```python
from build123d import *

# Parameters (mm, degrees)
SKETCH_W              = 18.5
SKETCH_H              = 18.5
SKETCH_R              = 8.15
PAD_DEPTH             = 4
SKETCH001_W           = 18.5
SKETCH001_H           = 18.5
PAD001_DEPTH          = 3
SKETCH002_R           = 9.25
SKETCH003_R           = 5.4
SKETCH005_R           = 5.4
PAD002_DEPTH          = 2
CHAMFER_SIZE          = 1.5
CHAMFER001_SIZE       = 1.5
POCKET_DEPTH          = 99.630527
POLARPATTERN_COUNT    = 4
SKETCH007_R           = 4.4
SKETCH008_R           = 5.4
SKETCH009_R           = 5.4
PAD003_DEPTH          = 7
SKETCH010_R           = 4.4
POCKET001_DEPTH       = 3
SKETCH011_W           = 1.7
SKETCH011_H           = 3
POCKET002_DEPTH       = 114.093887
POLARPATTERN001_COUNT = 5


with BuildPart() as part:
    # Sketch → Pad (new body)
    with BuildSketch(Plane.XY):
        Rectangle(SKETCH_W, SKETCH_H)
        Circle(SKETCH_R, mode=Mode.SUBTRACT)
    extrude(amount=PAD_DEPTH)

    # Sketch001 (on Face7 of Pad) → Pad001 (join)
    with BuildSketch(Plane.XY.offset(4)):
        Rectangle(SKETCH001_W, SKETCH001_H)
    extrude(amount=PAD001_DEPTH)

    # Sketch002 (on Face10 of Pad001) → AdditiveLoft section 0
    with BuildSketch(Plane.XY.offset(7)):
        Circle(SKETCH002_R)
    # Sketch003 (on Face10 of Pad001) → AdditiveLoft section 1
    with BuildSketch(Plane.XY.offset(29)):
        Circle(SKETCH003_R)
    loft()

    # Sketch005 (on Face17 of AdditiveLoft) → Pad002 (join)
    with BuildSketch(Plane.XY.offset(29)):
        Circle(SKETCH005_R)
    extrude(amount=PAD002_DEPTH)

    # Chamfer
    chamfer_edges = [part.edges().sort_by_distance(p)[0] for p in [
        (-9.25, -9.25, 5.5),
        (-9.25, -9.25, 2),
        (9.25, -9.25, 5.5),
        (9.25, -9.25, 2),
        (9.25, 9.25, 2),
        (9.25, 9.25, 5.5),
        (-9.25, 9.25, 5.5),
        (-9.25, 9.25, 2),
    ]]
    chamfer(chamfer_edges, length=CHAMFER_SIZE)

    # Chamfer001
    chamfer001_edges = [part.edges().sort_by_distance(p)[0] for p in [
        (8.5, -8.5, 7),
        (-8.5, -8.5, 7),
        (-8.5, 8.5, 7),
        (8.5, 8.5, 7),
    ]]
    chamfer(chamfer001_edges, length=CHAMFER001_SIZE)

    # Sketch006 (on Face19 of Chamfer001) → Pocket (cut, through all)
    with BuildSketch(Plane.YZ.offset(9.25)):
        Polygon((0, 29), (-2.7, 7), (2.7, 7), align=None)
    pocket = extrude(amount=-POCKET_DEPTH, mode=Mode.SUBTRACT)

    # PolarPattern: Pocket ×4 about axis
    polarpattern_axis = Axis((0, 0, 0), (0, 0, 1))
    for i in range(1, POLARPATTERN_COUNT):
        add(pocket.rotate(polarpattern_axis, i * 360 / POLARPATTERN_COUNT), mode=Mode.SUBTRACT)

    # Sketch007 (on Face47 of PolarPattern) → AdditiveLoft001 section 0
    with BuildSketch(Plane.XY.offset(31)):
        Circle(SKETCH007_R)
    # Sketch008 → AdditiveLoft001 section 1
    with BuildSketch(Plane.XY.offset(33)):
        Circle(SKETCH008_R)
    loft()

    # Sketch009 (on Face56 of AdditiveLoft001) → Pad003 (join)
    with BuildSketch(Plane.XY.offset(33)):
        Circle(SKETCH009_R)
    extrude(amount=PAD003_DEPTH)

    # Sketch010 (on Face57 of Pad003) → Pocket001 (cut)
    with BuildSketch(Plane.XY.offset(40)):
        Circle(SKETCH010_R)
    extrude(amount=-POCKET001_DEPTH, mode=Mode.SUBTRACT)

    # Sketch011 (on Face26 of Pocket001) → Pocket002 (cut, through all)
    with BuildSketch(Plane.YZ.offset(9.25)):
        with Locations((0, 38.5)):
            Rectangle(SKETCH011_W, SKETCH011_H)
    pocket002 = extrude(amount=-POCKET002_DEPTH, mode=Mode.SUBTRACT)

    # PolarPattern001: Pocket002 ×5 about axis
    polarpattern001_axis = Axis((0, 0, 0), (0, 0, 1))
    for i in range(1, POLARPATTERN001_COUNT):
        add(pocket002.rotate(polarpattern001_axis, i * 360 / POLARPATTERN001_COUNT), mode=Mode.SUBTRACT)


solid = part.part
```
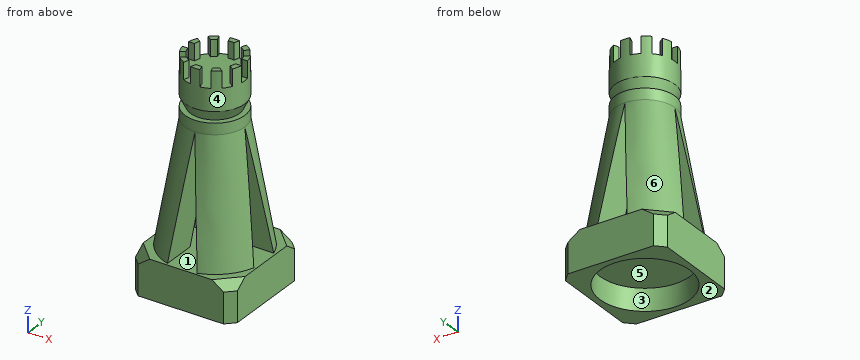
Could you check a few things on this model? Use its own coordinates, in mm. Face numbers are marked on the shaded views. A direction names the side the tool comes from. Coordinates: 2 decimals unless noted, no trailing zeros. Write each loop counter-clockwise with the first axis right and the second up, starting at its lowest first coordinate (ties: lowest second). Pieces come first, ordered by that corner, then holes. Notation, with made-up numbers: (-8, -12) -> (40, -12) arc R15 cw to (40, 3) -> close; hole circle Ø6 at (6, -25). An arc over 180 degrees is marked (long way). Return JSON: item names as keys, results as strings.
(1) Imagine slicing it at B-B, the plane z = 7.5. Please give me the cut outline in (x, y) (1 decimal), then the cut area to 3 significant figures.
Numbers:
{"outline": "(-8.8, -2.6) arc R9.2 ccw to (-2.6, -8.8) -> (-2.6, -2.6) -> close; (-8.8, 2.6) -> (-2.6, 2.6) -> (-2.6, 8.8) arc R9.2 ccw to start; (2.6, -8.8) arc R9.2 ccw to (8.8, -2.6) -> (2.6, -2.6) -> close; (2.6, 2.6) -> (8.8, 2.6) arc R9.2 ccw to (2.6, 8.8) -> close", "area": "101 mm2"}
(2) Imagine slicing it at A-A, the plane z = 28.5. Please give me the cut outline in (x, y) (1 decimal).
Numbers:
{"outline": "(-5.5, -0.1) arc R5.5 ccw to (-0.1, -5.5) -> (-0.1, -0.1) -> close; (-5.5, 0.1) -> (-0.1, 0.1) -> (-0.1, 5.5) arc R5.5 ccw to start; (0.1, -5.5) arc R5.5 ccw to (5.5, -0.1) -> (0.1, -0.1) -> close; (0.1, 0.1) -> (5.5, 0.1) arc R5.5 ccw to (0.1, 5.5) -> close"}
(3) I need wall thicknesses on L1, parallel to Y at x = 0, z = 2.65; L2, parallel to X at y = -4, z = 8; L3, parallel to X at y = 3.75, z = 18. Which ranges of each line are inside material? Lowest first, please.
Numbers:
{"L1": "y = -9.25 to -8.15, 8.15 to 9.25", "L2": "x = -8.15 to -2.58, 2.58 to 8.15", "L3": "x = -6.29 to -1.35, 1.35 to 6.29"}
(4) We'd pull the mould along Y, two halves only. Please class the marked faces 1, 2, 3 and 4: +Y half, -Y half, draft (parallel to the pull), parting line (faces both ways), or undercut.
Numbers:
{"face 1": "undercut", "face 2": "draft", "face 3": "undercut", "face 4": "parting line"}
(5) Which directions (+Z, -Z, +X, -X, +Y, -Y) give clear straight access to the entire face, cutting with the end or side of a thin tool? Please do the marked faces 5 and 6.
Numbers:
{"face 5": "-Z", "face 6": "+Z, -X, +Y"}
(6) I'm going to push flat-ended pins straight in: pin 1 (2 mm diameter, centred on y = 5, z = 32, fed in from +X); pin 2 (3 mm diameter, centred on y = -1, z = 17.5, fed in from +X); pin 3 (1 mm diameter, centred on x = 1.5, y = 5, fed in from -Z). Where does each tip first touch, or does it pass through?
Numbers:
{"pin 1": "stops at x = 3.07", "pin 2": "stops at x = 7.49", "pin 3": "stops at z = 4"}
